Design review of the part built by this model. Coordinates are the model's own, in mm. Face numbers are marked on the shaded views. A direction names the side the tool comes from. Give positions to 0.01 mm unless a question says otherwise; leave off trailing zeros. Write each loop counter-clockwise with the first axis right and the second up, starting at its lowest first coordinate (ties: lowest second). Pieces come first, ordered by that corner, then holes. Notation, with made-up numbers: (8.25, 16) -> (28.25, 16) arc R22 cw to (28.25, 34) -> close; hole circle Ø3 at (-18, -14.5). An arc over 180 degrees is marked (long way). Use CSV: the item, a comma, the result in double quotes.
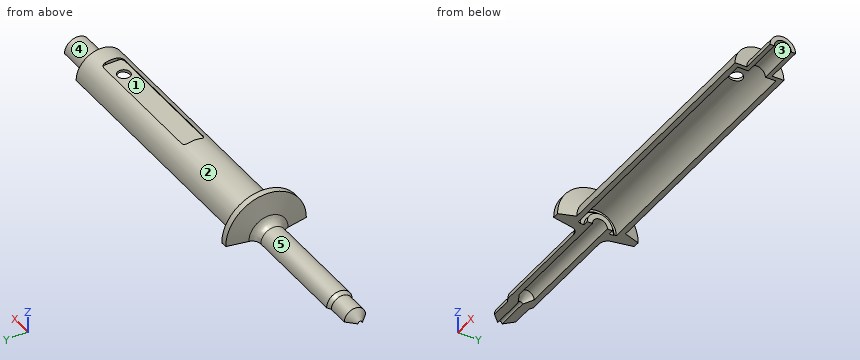
```python
from build123d import *

# Parameters (mm, degrees)
SKETCH005_W      = 32
SKETCH005_H      = 5
PAD002_DEPTH     = 10
FILLET_R         = 1
FILLET001_R      = 1
FILLET002_R      = 1
FILLET003_R      = 1
REVOLUTION_ANGLE = 180
SKETCH006_R      = 1.5
POCKET_DEPTH     = 5
FILLET004_R      = 2


with BuildPart() as obj1:
    # Sketch005 → Pad002 (new body)
    with BuildSketch(Plane.XY):
        with Locations((45, 0)):
            Rectangle(SKETCH005_W, SKETCH005_H)
    extrude(amount=PAD002_DEPTH)

    # Fillet
    fillet_edges = [obj1.edges().sort_by_distance(p)[0] for p in [
        (29, -2.5, 5),
    ]]
    fillet(fillet_edges, radius=FILLET_R)

    # Fillet001
    fillet001_edges = [obj1.edges().sort_by_distance(p)[0] for p in [
        (29, 2.5, 5),
    ]]
    fillet(fillet001_edges, radius=FILLET001_R)

    # Fillet002
    fillet002_edges = [obj1.edges().sort_by_distance(p)[0] for p in [
        (61, -2.5, 5),
    ]]
    fillet(fillet002_edges, radius=FILLET002_R)

    # Fillet003
    fillet003_edges = [obj1.edges().sort_by_distance(p)[0] for p in [
        (61, 2.5, 5),
    ]]
    fillet(fillet003_edges, radius=FILLET003_R)


with BuildPart() as obj1_1:
    # Body006 placement: moved
    add(obj1.part.moved(Location((0, 0, 5))))


with BuildPart() as half:
    # Sketch → Revolution (revolve)
    with BuildSketch(Plane.XY):
        Polygon((-34.657143, 0.5), (-32.657143, 2.5), (-27.657143, 2.5), (-26.657143, 3), (0.342857, 3), (1.592857, 9.5), (3.092857, 9.5), (4.342857, 5.75), (65.342857, 5.75), (65.342857, 3), (74.342857, 3), (74.342857, 2), (64.342857, 2), (64.342857, 4.5), (2.842015, 4.5), (2.842015, 3.942434), (2.64252, 3.942434), (2.64252, 3), (3.894188, 3), (3.894188, 1.75), (-24.320252, 1.75), (-26.820252, 0.5), align=None)
    revolve(axis=Axis((0, 0, 0), (1, 0, 0)), revolution_arc=REVOLUTION_ANGLE)

    # Boolean002: cut obj1
    add(obj1_1.part, mode=Mode.SUBTRACT)

    # Sketch006 (on Face33 of Boolean002) → Pocket (cut)
    with BuildSketch(Plane.XY.offset(5)):
        with Locations((56.342857, 0)):
            Circle(SKETCH006_R)
    extrude(amount=-POCKET_DEPTH, mode=Mode.SUBTRACT)

    # Fillet004
    fillet004_edges = [half.edges().sort_by_distance(p)[0] for p in [
        (0.342857, 0, 3),
    ]]
    fillet(fillet004_edges, radius=FILLET004_R)


solid = half.part
```
(1) For line 1 along X through (y, z) = (0, 4.65); line 2 along X through (y, z) = (0, 4.6); line 3 along Y through (x, z) = (-22, 1), list the stretches that pass through material, from the lowest coordinate up. Write a range as [from, to].
Established:
line 1,"x = [0.66, 54.84], [57.84, 65.34]"
line 2,"x = [0.65, 54.84], [57.84, 65.34]"
line 3,"y = [-2.83, -1.44], [1.44, 2.83]"
(2) Clearance check with flat-ended pins moving along their axes: pin 1 (2 mm diameter, centred on x = 38, z = 5, fed in from -Y); pin 2 (2 mm diameter, centred on y = -2, z = 3, fed in from +X); pin 3 (1.5 mm diameter, centred on x = 63, y = 3, fed in from +Z); pin 4 (5 mm diameter, centred on y = 4, z = 7, fed in from +X). State where each tip first meets the part, or that it passes through.
Established:
pin 1,"stops at y = -4.13"
pin 2,"stops at x = 74.34"
pin 3,"stops at z = 5.29"
pin 4,"stops at x = 65.34"
(3) Take a section at C-C (x = 13). Write out the cut boundary in (y, z), then the cut area to 3 significant figures.
Established:
outline,"(-5.75, 0) -> (-4.5, 0) arc R4.5 cw to (4.5, 0) -> (5.75, 0) arc R5.75 ccw to start"
area,"20.1 mm2"
(4) Take a section at A-A (x = 37.5). Write out the cut boundary in (y, z).
Established:
outline,"(-5.75, 0) -> (-4.5, 0) arc R4.5 cw to (4.5, 0) -> (5.75, 0) arc R5.75 ccw to (2.5, 5.18) -> (2.5, 5) -> (-2.5, 5) -> (-2.5, 5.18) arc R5.75 ccw to start"
(5) Take a section at B-B (x = -7.5). Write out the cut boundary in (y, z), then the cut area to 3 significant figures.
Established:
outline,"(-3, 0) -> (-1.75, 0) arc R1.75 cw to (1.75, 0) -> (3, 0) arc R3 ccw to start"
area,"9.33 mm2"
(6) Mouldability with a two-part tool opening along Y and no side actions: class the marked faces 1 and 2 as +Y half, -Y half, draft (parallel to the pull), parting line (faces both ways), or undercut.
Established:
face 1,"undercut"
face 2,"parting line"
(7) Tool access review of the marked faces 3, 4 and 5: name each direction out of +Z, -Z, +X, -X, +Y, -Y from which nothing blocks a thin tool from reaching the whole face with its end or side.
Established:
face 3,"-Z, +X"
face 4,"+Z, +X"
face 5,"+Z, -X"
